CAD build for the part. Positions are in the model's coordinates, mm. A direction names the side the tool comes from. Give positions to 0.01 mm unless a question says otherwise; leave off trailing zeros. Order: outer loops, then holes, each group sorted by start corner. A loop starts at its lowest first (then second) coordinate and runs counter-clockwise, first axis right, second up. Notation, with made-up numbers: M 27,43 L 78,43 A13 cw 78,51 Z; hole C 43,-27 d8. An arc over 180 degrees is marked long. Put each result on its own line as item: value. Start each with the question number.
1) Two-plate mould, pull along X, no slides. Class faces 1 (the face through (3.233, 9.106, 1.341)), 2 (the face through (2.5, -10, 0)), 3 (the face through (2, -10, 0)), 4 (the face through (0, 16.3, 2)): released by +X, released by -X, zero draft, split by the parting line, or undercut.
2) Pin check, flat tips, straight feed: pin 1 (3.5 mm diameter, centred on y = -11.5, z = -0.5, fed in from -X); pin 2 (0.6 mm diameter, centred on x = 2.5, y = -10.5, fed in from +Z); pin 3 (2.5 mm diameter, centred on y = -12.5, z = 0, fed in from +X). Stop position of each tip, or through.
3) Cut at A-A (y = -8.5). Write the cut outline in (x, z).
4) Tool access for faces 5 (the face through (2.2, 6, 3.3)), 6 (the face through (-2, -10, 0)), 7 (the face through (2.285, -3.944, 3.584)): list every direction of +Z, -Z, +X, -X, +Y, -Y with a clear straight run to the whole face (end or side of a thin tool).
5) Cut at C-C (x = 0). Write the cut outline in (y, z), and give its area (3 significant figures).
6) Drill centre lines: line 1 (Y direction, x = 3, z = -1.75); line 2 (Y direction, x = 3.5, z = 0.75); line 3 (Y direction, x = 0.75, z = 0.5). Where is each one in solid material? Low to high. Write a range as [from, to].
7) Cut at B-B (z = 0). Give the number of separate pieces and of enclosed holes in the cut face, and give its area (3 significant figures).
8) Cut at D-D (y = 4). Write the cut outline in (x, z).
```python
from build123d import *

# Parameters (mm, degrees)
ESBO_O1_R                = 5
RESSALTO_EXTRUS_O1_DEPTH = 6
ESBO_O2_R                = 4.25
RESSALTO_EXTRUS_O2_DEPTH = 8
ESBO_O3_W                = 0.5
ESBO_O3_H                = 3
RESSALTO_EXTRUS_O3_DEPTH = 6
ESBO_O4_W                = 1.442967266
ESBO_O4_H                = 2.423445024
CORTE_EXTRUS_O1_DEPTH    = 8.5
ESBO_O5_R                = 3.5
RESSALTO_EXTRUS_O4_DEPTH = 6.3
ESBO_O6_R                = 1.75
RESSALTO_EXTRUS_O5_DEPTH = 4
ESBO_O7_R                = 5
RESSALTO_EXTRUS_O6_DEPTH = 6.5
FILETE1_R                = 1


with BuildPart() as part:
    # Esboço1 → Ressalto-extrusão1 (new body)
    with BuildSketch(Plane(origin=(0, 0, 0), x_dir=(1, 0, 0), z_dir=(0, 1, 0))):
        Circle(ESBO_O1_R)
    extrude(amount=RESSALTO_EXTRUS_O1_DEPTH)

    # Esboço2 → Ressalto-extrusão2 (add)
    with BuildSketch(Plane.XZ):
        Circle(ESBO_O2_R)
    extrude(amount=RESSALTO_EXTRUS_O2_DEPTH)

    # Esboço3 → Ressalto-extrusão3 (add)
    with BuildSketch(Plane.XZ.offset(8)):
        with Locations((2.25, 0)):
            Rectangle(ESBO_O3_W, ESBO_O3_H)
        with Locations((-2.25, 0)):
            Rectangle(ESBO_O3_W, ESBO_O3_H)
    extrude(amount=RESSALTO_EXTRUS_O3_DEPTH)

    # Esboço4 → Corte-extrusão1 (cut, through all)
    with BuildSketch(Plane.ZY.offset(2.5)):
        with Locations((-0.007097641, -12.050464305)):
            Rectangle(ESBO_O4_W, ESBO_O4_H)
    extrude(amount=-CORTE_EXTRUS_O1_DEPTH, mode=Mode.SUBTRACT)

    # Esboço5 → Ressalto-extrusão4 (add)
    with BuildSketch(Plane(origin=(0, 6, 0), x_dir=(1, 0, 0), z_dir=(0, 1, 0))):
        Circle(ESBO_O5_R)
    extrude(amount=RESSALTO_EXTRUS_O4_DEPTH)

    # Esboço6 → Ressalto-extrusão5 (add)
    with BuildSketch(Plane(origin=(0, 12.3, 0), x_dir=(1, 0, 0), z_dir=(0, 1, 0))):
        Circle(ESBO_O6_R)
    extrude(amount=RESSALTO_EXTRUS_O5_DEPTH)

    # Esboço7 → Ressalto-extrusão6 (add)
    with BuildSketch(Plane(origin=(0, 16.3, 0), x_dir=(1, 0, 0), z_dir=(0, 1, 0))):
        Circle(ESBO_O7_R)
    extrude(amount=RESSALTO_EXTRUS_O6_DEPTH)

    # Filete1
    filete1_edges = [part.edges().sort_by_distance(p)[0] for p in [
        (-5, 22.8, 0),
    ]]
    fillet(filete1_edges, radius=FILETE1_R)


solid = part.part
```
Solution:
1. face 1: split by the parting line
1. face 2: released by +X
1. face 3: undercut
1. face 4: zero draft
2. pin 1: x = -2.5
2. pin 2: z = 1.5
2. pin 3: x = 2.5
3. outline: M -2.5,-1.5 L -2,-1.5 L -2,1.5 L -2.5,1.5 Z; M 2,-1.5 L 2.5,-1.5 L 2.5,1.5 L 2,1.5 Z
4. face 5: none
4. face 6: +Z, -Z, -Y
4. face 7: -Y
5. outline: M -8,-4.25 L 0,-4.25 L 0,-5 L 6,-5 L 6,-3.5 L 12.3,-3.5 L 12.3,-1.75 L 16.3,-1.75 L 16.3,-5 L 21.8,-5 A1 ccw 22.8,-4 L 22.8,4 A1 ccw 21.8,5 L 16.3,5 L 16.3,1.75 L 12.3,1.75 L 12.3,3.5 L 6,3.5 L 6,5 L 0,5 L 0,4.25 L -8,4.25 Z
5. area: 251 mm²
6. line 1: [-8, 12.3], [16.3, 22.8]
6. line 2: [-8, 6], [16.3, 22.8]
6. line 3: [-8, 22.8]
7. separate pieces: 3
7. enclosed holes: 0
7. area: 254 mm²
8. outline: C 0,0 d10
